```python
from build123d import *

# Parameters (mm, degrees)
PAD002_DEPTH            = 36
SKETCH006_W             = 69.825363
SKETCH006_H             = 30
POCKET002_DEPTH         = 36.001
SKETCH007_R             = 5
POCKET003_DEPTH         = 36.001
SKETCH008_R             = 5
POCKET004_DEPTH         = 5
BODY002_ROLL_ANGLE      = -90.304991
BODY002_PITCH_ANGLE     = -3.775431
BODY002_PLACEMENT_ANGLE = -46.199273


with BuildPart() as part:
    # Sketch005 → Pad002 (new body)
    with BuildSketch(Plane.XY):
        with BuildLine():
            Line((-18, 0), (18, 0))
            Line((18, 0), (18, 50))
            ThreePointArc((18, 50), (0, 59.792689), (-18, 50))
            Line((-18, 50), (-18, 0))
        make_face()
    extrude(amount=PAD002_DEPTH)

    # Sketch006 (on Face2 of Pad002) → Pocket002 (cut, through all)
    with BuildSketch(Plane.YZ.offset(18)):
        with Locations((37.912681, 18)):
            Rectangle(SKETCH006_W, SKETCH006_H)
    extrude(amount=-POCKET002_DEPTH, mode=Mode.SUBTRACT)

    # Sketch007 (on Face5 of Pocket002) → Pocket003 (cut, through all)
    with BuildSketch(Plane.XY.offset(36)):
        with Locations((0, 49.623631)):
            Circle(SKETCH007_R)
    extrude(amount=-POCKET003_DEPTH, mode=Mode.SUBTRACT)

    # Sketch008 (on Face1 of Pocket003) → Pocket004 (cut)
    with BuildSketch(Plane.XZ):
        with Locations((0, 25)):
            Circle(SKETCH008_R)
    extrude(amount=-POCKET004_DEPTH, mode=Mode.SUBTRACT)


with BuildPart() as part_1:
    # Body002 roll: moved
    add(part.part.rotate(Axis((0, 0, 0), (1, 0, 0)), BODY002_ROLL_ANGLE))


with BuildPart() as part_2:
    # Body002 pitch: moved
    add(part_1.part.rotate(Axis((0, 0, 0), (0, 1, 0)), BODY002_PITCH_ANGLE))


with BuildPart() as part_3:
    # Body002 placement: moved
    add(part_2.part.moved(Location((-19.80148, -78.155877, 488.747301))).rotate(Axis((-19.80148, -78.155877, 488.747301), (0, 0, 1)), BODY002_PLACEMENT_ANGLE))


solid = part_3.part
```
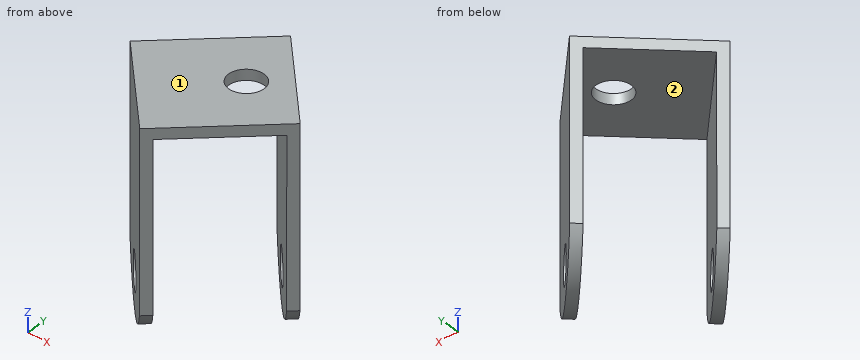
Could you check a few things on this model? Use its own coordinates, in mm. Face numbers are marked on the shaded views. Give positions to 0.01 mm unless a question says otherwise; leave off trailing zeros. Order: outer loops, then holes, each group sorted by start corner. A loop starts at its lowest first (then second) coordinate and runs counter-clockwise, first axis right, second up.
Q1. We'd pull the mould along X, two halves only. Please class the marked faces 1 and 2: +X half, -X half, draft (parallel to the pull), parting line (faces both ways), or undercut.
Q2. I'm going to push flat-ended pins straight in: P1, Ø8, axis at y = -53.5, z = 481, coming from the -X side; P2, Ø3, axis at x = 4, y = -67, coming from the +Z side; P3, Ø12, axis at y = -54, z = 468.5, coming from the +X side; P4, Ø1, axis at x = -4, y = -59.5, coming from the -Z side. Where does each tip first touch, or does it pass through?
Q3. Suppose I cut it at A-A, the plane z = 480. Write out the boundary of the cut face in (x, y), and give its area (3 significant figures).
Q4. If I drill on line 1 along X through (y, z) = (-68, 471.5); line 2 along Y through (x, z) = (-1, 442); line 3 along X through (y, z) = (-68, 460), over which ranges is the centre line in solid material (lowest first)?
Solution:
1. face 1: -X half
1. face 2: undercut
2. P1: stops at x = -21.78
2. P2: stops at z = 489.27
2. P3: stops at x = 12.51
2. P4: passes through
3. outline: (-31.92, -65.58) - (-6.95, -91.63) - (-4.79, -89.55) - (-29.75, -63.5) - close; (-8.1, -42.74) - (16.86, -68.79) - (19.03, -66.71) - (-5.93, -40.66) - close
3. area: 216 mm2
4. line 1: x = -29.66 to -25.51, 16.05 to 18.5
4. line 2: y = -50.44 to -46.1
4. line 3: x = -29.75 to -25.59, 15.96 to 19.59
